from build123d import *

# Parameters (mm, degrees)
SKETCH1_R           = 2.25
BOSS_EXTRUDE1_DEPTH = 12.7
FILLET1_R           = 6.35
FILLET3_R           = 6.35
FILLET4_R           = 1
CUT_EXTRUDE1_REACH  = 121.755
SKETCH2_R           = 2.25


with BuildPart() as part:
    # Sketch1 → Boss-Extrude1 (new body)
    with BuildSketch(Plane(origin=(0, 0, 0), x_dir=(0, 0, -1), z_dir=(1, 0, 0))):
        with BuildLine():
            Line((-25.4, 87.319743879), (-25.4, 11.3))
            Line((-25.4, 11.3), (-50.8, 11.3))
            Line((-50.8, 11.3), (-50.8, 4.95))
            Line((-50.8, 4.95), (-25.4, 4.95))
            Line((-25.4, 4.95), (-2.706927177, -5.744131375))
            ThreePointArc((-2.706927177, -5.744131375), (5.744131375, -2.706927177), (2.706927177, 5.744131375))
            Line((2.706927177, 5.744131375), (-12.7, 13.004659934))
            Line((-12.7, 13.004659934), (-12.7, 92.580256121))
            Line((-12.7, 92.580256121), (-30.909871939, 110.790128061))
            ThreePointArc((-30.909871939, 110.790128061), (-39.890128061, 110.790128061), (-39.890128061, 101.809871939))
            Line((-39.890128061, 101.809871939), (-25.4, 87.319743879))
        make_face()
        with Locations((-35.4, 106.3)):
            Circle(SKETCH1_R, mode=Mode.SUBTRACT)
        Circle(SKETCH1_R, mode=Mode.SUBTRACT)
    extrude(amount=BOSS_EXTRUDE1_DEPTH)

    # Fillet1
    fillet1_edges = [part.edges().sort_by_distance(p)[0] for p in [
        (6.35, 4.95, 25.4),
        (6.35, 87.319743879, 25.4),
        (6.35, 92.580256121, 12.7),
        (6.35, 13.004659934, 12.7),
    ]]
    fillet(fillet1_edges, radius=FILLET1_R)

    # Fillet3
    fillet3_edges = [part.edges().sort_by_distance(p)[0] for p in [
        (0, 8.125, 50.8),
        (12.7, 8.125, 50.8),
    ]]
    fillet(fillet3_edges, radius=FILLET3_R - 0.0001)  # a hair under: the kernel refuses the full size

    # Fillet4
    fillet4_edges = [part.edges().sort_by_distance(p)[0] for p in [
        (12.7, -2.706927177, -5.744131375),
        (0, 11.3, 34.92505),
        (0, 47.994743879, 25.4),
        (0, 110.790128061, 39.890128061),
        (0, 102.615128061, 22.734871939),
        (0, -2.706927177, -5.744131375),
        (6.35, 11.3, 25.4),
        (12.7, 102.615128061, 22.734871939),
        (12.7, 110.790128061, 39.890128061),
        (0, -0.7, 13.410633407),
        (12.7, -0.7, 13.410633407),
        (12.7, 47.994743879, 25.4),
        (0, 53.490994951, 12.7),
        (12.7, 53.490994951, 12.7),
        (0, 8.515994951, 3.175),
        (12.7, 8.515994951, 3.175),
        (12.7, 11.3, 34.92505),
        (0, 95.494743879, 33.575),
        (0, 92.380039796, 13.183364969),
        (12.7, 95.494743879, 33.575),
        (12.7, 92.380039796, 13.183364969),
        (0, 4.796681944, 25.434315884),
        (12.7, 4.796681944, 25.434315884),
        (0, 13.630996486, 11.712438232),
        (12.7, 13.630996486, 11.712438232),
        (0, 87.119527553, 25.883364969),
        (12.7, 87.119527553, 25.883364969),
        (0, 4.95, 35.635683407),
        (12.7, 4.95, 35.635683407),
        (10.84015735, 4.95, 48.94015735),
        (1.85984265, 4.95, 48.94015735),
        (10.84015735, 11.3, 48.94015735),
        (1.85984265, 11.3, 48.94015735),
    ]]
    fillet(fillet4_edges, radius=FILLET4_R)

    # Sketch2 → Cut-Extrude1 (cut, up to next)
    with BuildSketch(Plane.XZ.offset(-4.95), mode=Mode.PRIVATE) as cut_extrude1_sk1:
        with Locations(Location((6.35, 31.75, 0), (0, 0, 270))):
            Circle(SKETCH2_R)
    cut_extrude1_tool1 = extrude(cut_extrude1_sk1.sketch, amount=-CUT_EXTRUDE1_REACH, mode=Mode.PRIVATE) & part.part
    # Sketch2 → Cut-Extrude1 (cut, up to next)
    with BuildSketch(Plane.XZ.offset(-4.95), mode=Mode.PRIVATE) as cut_extrude1_sk2:
        with Locations(Location((6.35, 44.45, 0), (0, 0, 270))):
            Circle(SKETCH2_R)
    cut_extrude1_tool2 = extrude(cut_extrude1_sk2.sketch, amount=-CUT_EXTRUDE1_REACH, mode=Mode.PRIVATE) & part.part
    add(cut_extrude1_tool1.solids().sort_by_distance((6.35, 4.95, 31.75))[0], mode=Mode.SUBTRACT)
    add(cut_extrude1_tool2.solids().sort_by_distance((6.35, 4.95, 44.45))[0], mode=Mode.SUBTRACT)


solid = part.part
Here's how the part is built. I have some questions about the finished solid (model axes, mm). Give positions to 0.01 mm unless a question says otherwise; leave off trailing zeros. Write each loop counter-clockwise with the first axis right and the second up, starting at its lowest first coordinate (ties: lowest second). Pieces come first, ordered by that corner, then holes. Notation, with made-up numbers: (-27, -37) -> (21, -37) arc R8 ccw to (21, -32) -> close; hole circle Ø1 at (87, 36). An arc over 180 degrees is marked (long way). Use one line per item in the form item = value. Start each with the question number.
1. If I drill on L1, parallel to Y at x = 1.75, z = 34.5; L2, parallel to Y at x = 4.5, z = 34; L3, parallel to X at y = 7, z = 31.75, over which ranges is the centre line in solid material (lowest first)?
2. Imagine slicing it at B-B on z = 35.4. State how many separate pieces and enclosed holes the cut face has, plus the area to 3 significant figures.
3. Imagine slicing it at A-A on y = 56. List the corners of the cut face in (x, z) for me.
4. Will these pins go through, and if not, where does the flat tip stop? pin 1 Ø1 at (x, y) = (7, 55) entering from -Z; pin 2 Ø5 at (x, z) = (6.35, 31.75) entering from -Y; pin 3 Ø4 at (x, y) = (6.5, 87.5) entering from +Z.
5. Thinking about a two-plate mould opening in Y: for faces 1 (the face through (12.399, 95.608, 33.285)), 2 (the face through (0.301, 95.785, 33.462)), 3 (the face through (0, 49, 22)), 4 (the face through (6, 4.95, 38)), which applies, +Y half, -Y half, draft (parallel to the pull), parting line (faces both ways), or undercut?
Entries:
q1.L1 = 4.95 to 11.3, 96.42 to 104.24, 108.36 to 112.59
q1.L2 = 4.95 to 11.3, 95.92 to 104.54, 108.06 to 112.49
q1.L3 = 0 to 4.1, 8.6 to 12.7
q2.separate_pieces = 3
q2.enclosed_holes = 0
q2.area = 216 mm²
q3.outline = (0, 13.7) arc R1 ccw to (1, 12.7) -> (11.7, 12.7) arc R1 ccw to (12.7, 13.7) -> (12.7, 24.4) arc R1 ccw to (11.7, 25.4) -> (1, 25.4) arc R1 ccw to (0, 24.4) -> close
q4.pin_1 = 12.7
q4.pin_2 = 4.95
q4.pin_3 = 27.58
q5.face_1 = undercut
q5.face_2 = undercut
q5.face_3 = draft
q5.face_4 = -Y half
